Source: CAD feature listing. Evaluate the final solid. Frame: model axes, mm. A direction names the side the tool comes from. Coordinates: 2 decimals unless noted, no trailing zeros. Loops run counter-clockwise (first coordinate to the right, second up) from the corner with the lowest first, then second, coordinate; pieces in that order, holes last. Notation, with made-up numbers: (60.25, 20.25) - (92.25, 20.25) arc R20 cw to (92.25, 37.25) - close; hole circle Ø9 at (75.5, -13.5). An arc over 180 degrees is marked (long way). Use one line per item in the form item = value. Start each with the question number.
from build123d import *

# Parameters (mm, degrees)
BOSS_EXTRUDE1_DEPTH     = 15.9
SHELL1_START            = -14.7
SHELL1_DEPTH            = 13.5
CUT_EXTRUDE1_DEPTH      = 29.819656487
CUT_EXTRUDE1_DEPTH_BACK = 29.819656487
SKETCH3_W               = 8.5
SKETCH3_H               = 2.8
CUT_EXTRUDE2_START      = -1.2
CUT_EXTRUDE2_DEPTH      = 1.2
LPATTERN1_COUNT         = 2
LPATTERN1_PITCH         = 12.3
SKETCH5_W               = 11.1
SKETCH5_H               = 2.99
CUT_EXTRUDE5_DEPTH      = 0.8
SKETCH6_W               = 8.7
SKETCH6_H               = 0.59
BOSS_EXTRUDE2_DEPTH     = 1.1
SKETCH7_W               = 11.1
SKETCH7_H               = 1.1
CUT_EXTRUDE6_DEPTH      = 0.17
SKETCH8_W               = 0.5
SKETCH8_H               = 1.4
BOSS_EXTRUDE3_DEPTH     = 2.5
LPATTERN2_COUNT         = 2
LPATTERN2_PITCH         = 9


# Read off the part's stored shape, not the designer's step: Shell1
with BuildPart() as part:
    # Sketch2 → Boss-Extrude1 (new body)
    with BuildSketch(Plane(origin=(0, 0, 0), x_dir=(0, 0, -1), z_dir=(1, 0, 0))):
        with BuildLine():
            Line((-1.495, 0), (1.495, 0))
            Line((1.495, 0), (1.495, -22.355))
            ThreePointArc((1.495, -22.355), (0, -23.85), (-1.495, -22.355))
            Line((-1.495, -22.355), (-1.495, 0))
        make_face()
    extrude(amount=-BOSS_EXTRUDE1_DEPTH)

    # Shell1 outline → Shell1 (cut)
    with BuildSketch(Plane.YZ.offset(SHELL1_START)):
        with BuildLine():
            Line((-22.355, -0.295), (-22.355, -1.495))
            Line((-22.355, -1.495), (-1.2, -1.495))
            Line((-1.2, -1.495), (-1.2, 0.295))
            Line((-1.2, 0.295), (-22.355, 0.295))
            ThreePointArc((-22.355, 0.295), (-22.65, 0), (-22.355, -0.295))
        make_face()
    extrude(amount=SHELL1_DEPTH, mode=Mode.SUBTRACT)

    # Sketch3 → Cut-Extrude1 (cut, two sides: drawn at the far end of the back side and taken through both)
    with BuildSketch(Plane.XY.offset(1.495).offset(-CUT_EXTRUDE1_DEPTH_BACK)):
        with Locations((-7.95, -2.6)):
            Rectangle(SKETCH3_W, SKETCH3_H)
    extrude(amount=CUT_EXTRUDE1_DEPTH + CUT_EXTRUDE1_DEPTH_BACK, mode=Mode.SUBTRACT)

    # Sketch4 → Cut-Extrude2 (cut)
    with BuildSketch(Plane.ZY.offset(14.7).offset(CUT_EXTRUDE2_START)):
        with BuildLine():
            Line((1.495, -20.86), (-1.495, -20.86))
            Line((-1.495, -20.86), (-1.495, -22.355))
            ThreePointArc((-1.495, -22.355), (0, -23.85), (1.495, -22.355))
            Line((1.495, -22.355), (1.495, -20.86))
        make_face()
    cut_extrude2 = extrude(amount=CUT_EXTRUDE2_DEPTH, mode=Mode.SUBTRACT)

    # LPattern1: Cut-Extrude2 ×2
    with Locations(*[(i * LPATTERN1_PITCH, 0, 0) for i in range(1, LPATTERN1_COUNT)]):
        add(cut_extrude2, mode=Mode.SUBTRACT)

    # Sketch5 → Cut-Extrude5 (cut)
    with BuildSketch(Plane(origin=(0, 0, -1.495), x_dir=(-1, 0, 0), z_dir=(0, 0, -1))):
        with Locations((7.95, -22.355)):
            Rectangle(SKETCH5_W, SKETCH5_H)
    extrude(amount=-CUT_EXTRUDE5_DEPTH, mode=Mode.SUBTRACT)

    # Sketch6 → Boss-Extrude2 (add)
    with BuildSketch(Plane(origin=(0, 0, 0.295), x_dir=(-1, 0, 0), z_dir=(0, 0, -1))):
        Polygon((2.4, -20.86), (13.5, -20.86), (13.5, -23.85), (12.3, -23.85), (3.6, -23.85), (2.4, -23.85), align=None)
        with Locations((7.95, -22.355)):
            Rectangle(SKETCH6_W, SKETCH6_H, mode=Mode.SUBTRACT)
    extrude(amount=BOSS_EXTRUDE2_DEPTH)

    # Sketch7 → Cut-Extrude6 (cut)
    with BuildSketch(Plane.XZ.offset(23.85)):
        with Locations((-7.95, -0.255)):
            Rectangle(SKETCH7_W, SKETCH7_H)
    extrude(amount=-CUT_EXTRUDE6_DEPTH, mode=Mode.SUBTRACT)

    # Sketch8 → Boss-Extrude3 (add)
    with BuildSketch(Plane(origin=(0, 0, 0.295), x_dir=(-1, 0, 0), z_dir=(0, 0, -1))):
        with Locations((3.45, -1.9)):
            Rectangle(SKETCH8_W, SKETCH8_H)
    boss_extrude3 = extrude(amount=BOSS_EXTRUDE3_DEPTH)

    # LPattern2: Boss-Extrude3 ×2
    with Locations(*[(-i * LPATTERN2_PITCH, 0, 0) for i in range(1, LPATTERN2_COUNT)]):
        add(boss_extrude3)


solid = part.part
(1) Cut plane C-C, the plane y = -20. Output: boundary loops of the cut face in (x, z) (3 decimals), plus the area to 3 significant figures.
(2) Access query for faces 1 (the face through (-8, -23.68, 0)), 2 (the face through (-3.7, -2, 0)), 3 (the face through (-14, -1.2, -1)), 4 (the face through (-14, -20.86, 1)). Directions: +Z, -Z, +X, -X, +Y, -Y. A direction counts if a zero-diameter tool reaches every point of the face in a straight line with its end or side. Return the directions, or none.
(3) Mould query, pull axis X, two halves, no side actions, for faces 5 (the face through (0, -12, 0)), 6 (the face through (-2.4, -22, 0)), 7 (the face through (-15.9, -12, 0)), 8 (the face through (-8, -11, 1.495)). Classes: +X half, -X half, draft (parallel to the pull), parting line (faces both ways), or undercut.
(4) Cut plane B-B, the plane x = -9.75. Output: boundary loops of the cut face in (y, z) (3 decimals).
(5) Material intervals for line 1 (X direction, y = -21.75, z = 1.3); line 2 (X direction, y = -2.5, z = 0.15); line 3 (Y direction, x = -8.5, z = 0.05), sorted ascending.
(6) Contact query for flat-ended pins moving along their axis: pin 1 (5 mm diameter, centred on x = -11, y = -8, fed in from -Z) (3 decimals); pin 2 (1.5 mm diameter, centred on x = -11.5, z = -1.5, fed in from -Y); pin 3 (0.9 mm diameter, centred on x = -6, z = 0, fed in from -Y). Output: stop coordinate, or through.
(7) Cut plane D-D, the plane z = -1.1. Output: boundary loops of the cut face in (x, y).
(8) Cut plane A-A, the plane z = 0. Output: boundary loops of the cut face in (x, y).
Recorded:
q1.outline = (-15.9, -1.495) - (-14.7, -1.495) - (-14.7, 0.295) - (-1.2, 0.295) - (-1.2, -1.495) - (0, -1.495) - (0, 1.495) - (-15.9, 1.495) - close
q1.area = 23.4 mm²
q2.face_1 = -Z, -Y
q2.face_2 = +Z, -Z
q2.face_3 = -Z
q2.face_4 = +Z, -Z, -Y
q3.face_5 = +X half
q3.face_6 = undercut
q3.face_7 = -X half
q3.face_8 = draft
q4.outline = (-23.821, 0.295) - (-23.68, 0.295) - (-23.68, -0.805) - (-22.65, -0.805) - (-22.65, -0.695) - (-22.355, -0.695) - (-22.355, -0.295) arc R0.295 cw to (-22.355, 0.295) - (-22.06, 0.295) - (-22.06, -0.805) - (-20.86, -0.805) - (-20.86, 0.295) - (-4, 0.295) - (-4, 1.495) - (-22.355, 1.495) arc R1.495 ccw to start; (-1.2, -1.495) - (0, -1.495) - (0, 1.495) - (-1.2, 1.495) - close
q5.line_1 = -15.9 to -14.7, -13.5 to -2.4, -1.2 to 0
q5.line_2 = -15.9 to -14.7, -12.7 to -12.2, -3.7 to -3.2, -1.2 to 0
q5.line_3 = -23.68 to -22.65, -22.06 to -20.86, -1.2 to 0
q6.pin_1 = 0.295
q6.pin_2 = -23.68
q6.pin_3 = -23.82
q7.outline = (-15.9, -23.37) - (-14.7, -23.37) - (-14.7, -1.2) - (-12.7, -1.2) - (-12.7, -2.6) - (-12.2, -2.6) - (-12.2, -1.2) - (-3.7, -1.2) - (-3.7, -2.6) - (-3.2, -2.6) - (-3.2, -1.2) - (-1.2, -1.2) - (-1.2, -23.37) - (0, -23.37) - (0, 0) - (-15.9, 0) - close
q8.outline = (-15.9, -23.85) - (-14.7, -23.85) - (-14.7, -1.2) - (-12.7, -1.2) - (-12.7, -2.6) - (-12.2, -2.6) - (-12.2, -1.2) - (-3.7, -1.2) - (-3.7, -2.6) - (-3.2, -2.6) - (-3.2, -1.2) - (-1.2, -1.2) - (-1.2, -23.85) - (0, -23.85) - (0, 0) - (-15.9, 0) - close; (-13.5, -23.68) - (-2.4, -23.68) - (-2.4, -20.86) - (-13.5, -20.86) - close; hole (-12.3, -22.65) - (-3.6, -22.65) - (-3.6, -22.06) - (-12.3, -22.06) - close
